```python
from build123d import *

# Parameters (mm, degrees)
SKETCH1_W             = 96
SKETCH1_H             = 12
BOSS_EXTRUDE1_DEPTH   = 30
SKETCH1_3_R           = 7.5
BOSS_EXTRUDE2_DEPTH   = 6
BOSS_EXTRUDE3_DEPTH   = 20
BOSS_EXTRUDE4_DEPTH   = 7
F_8_0MM_DOWEL_HOLE1_D = 8
F_8_0MM_DOWEL_HOLE2_D = 8


with BuildPart() as part:
    # Sketch1 → Boss-Extrude1 (new body)
    with BuildSketch(Plane.XY):
        with Locations((0, 6)):
            Rectangle(SKETCH1_W, SKETCH1_H)
    extrude(amount=BOSS_EXTRUDE1_DEPTH)

    # Sketch1_3 → Boss-Extrude2 (add)
    with BuildSketch(Plane.XY):
        with BuildLine():
            ThreePointArc((-15, 56), (0, 41), (15, 56))
            Line((15, 56), (15, 46))
            Line((15, 46), (27, 46))
            ThreePointArc((27, 46), (34.864825613, 27.37239229), (48, 12))
            Line((48, 12), (-48, 12))
            ThreePointArc((-48, 12), (-34.864825613, 27.37239229), (-27, 46))
            Line((-27, 46), (-15, 46))
            Line((-15, 46), (-15, 56))
        make_face()
        with Locations((0, 27)):
            Circle(SKETCH1_3_R, mode=Mode.SUBTRACT)
    extrude(amount=BOSS_EXTRUDE2_DEPTH)

    # Sketch1_4 → Boss-Extrude3 (add)
    with BuildSketch(Plane.XY):
        Polygon((-27, 46), (-15, 46), (-15, 56), (-15, 66), (-27, 66), align=None)
        Polygon((15, 46), (15, 56), (15, 66), (27, 66), (27, 46), align=None)
    extrude(amount=BOSS_EXTRUDE3_DEPTH)

    # Sketch2 → Boss-Extrude4 (add)
    with BuildSketch(Plane(origin=(-15, 0, 0), x_dir=(0, 0, -1), z_dir=(1, 0, 0))):
        with BuildLine():
            Line((-20, 46), (-6, 46))
            Line((-6, 46), (-6, 12))
            Line((-6, 12), (-30, 12))
            ThreePointArc((-30, 12), (-22.675193853, 28.316233486), (-20, 46))
        make_face()
    boss_extrude4 = extrude(amount=-BOSS_EXTRUDE4_DEPTH)

    # Mirror1: Boss-Extrude4 across plane
    add(boss_extrude4.mirror(Plane(origin=(0, 0, 0), x_dir=(0, 0, 1), z_dir=(1, 0, 0))))

    # 8.0mm Dowel Hole1 (through all)
    with Locations(Plane(origin=(-27, 56, 10), x_dir=(0, -1, 0), z_dir=(-1, 0, 0))):
        with Locations((0, 0)):
            Hole(F_8_0MM_DOWEL_HOLE1_D / 2)

    # 8.0mm Dowel Hole2 (through all)
    with Locations(Plane(origin=(-32.5, 12, 18), x_dir=(0, 0, 1), z_dir=(0, 1, 0))):
        with Locations((0, 0), (0.381139368, 64.99888255)):
            Hole(F_8_0MM_DOWEL_HOLE2_D / 2)


solid = part.part
```
Can you work these out from the model? Positions are in its coordinate system, mm. A direction names the side the tool comes from. Round coordinates to 2 decimals unless told otherwise and drop trailing zeros. Loops run counter-clockwise (first coordinate to the right, second up) from the corner with the lowest first, then second, coordinate; pieces in that order, holes last. Notation, with made-up numbers: M 23.25,11 L 71.25,11 A19 ccw 71.25,19 Z; hole C -15.5,-30.5 d6. An arc over 180 degrees is marked long. Answer as a JSON object with one key per item and string values. Group by question number.
Q1. Imagine slicing it at B-B, the plane x = 0. Please give me the cut outline in (y, z), then the cut area to 3 significant figures.
Q2. We'd pull the mould along Y, two halves only. Please class faces 1 (the flat face through (0, 12, 18)), 2 (the flat face through (-22, 29, 15)), 3 (the flat face through (-1, 0, 15)), 4 (the flat face through (-21, 56, 20)): +Y half, -Y half, draft (parallel to the pull), parting line (faces both ways), or undercut.
Q3. Imagine slicing it at A-A, the plane z = 10. Please give me the cut outline in (x, y), then the cut area to 3 significant figures.
Q4. Will these pins go through, and if not, where does the flat tip stop? pin 1 (13 mm diameter, centred on x = 22, y = 58, fed in from +Z); pin 2 (1.5 mm diameter, centred on x = -34, z = 13, fed in from +Y); pin 3 (7 mm diameter, centred on y = 27, z = 16.5, fed in from +X).
Q5. Imagine slicing it at C-C, the plane y = 31. Please give me the cut outline in (x, z).
Q6. On a 3-axis mill with a long thin cutter (end or side, diameter ignored), from which of +Z, -Z, +X, -X, +Y, -Y can I reach the whole of each face in a straight line? I mean faces 5 (the cylindrical face through (0, 41, 3)), 6 (the flat face through (4, 34, 6)), 7 (the flat face through (-38, 12, 18)), 8 (the flat face through (21, 56, 20)). Say none if no direction works.
Q7. Please list where these lines run through material, in increasing order: L1, parallel to Y at x = -20.75, z = 10; L2, parallel to X at y = 19, z = 14; L3, parallel to X at y = 10, z = 20.5.
Q8. Imagine slicing it at D-D, the plane y = 5. Please give me the cut outline in (x, z).
Findings:
{
 "1": {"outline": "M 0,0 L 19.5,0 L 19.5,6 L 12,6 L 12,30 L 0,30 Z; M 34.5,0 L 41,0 L 41,6 L 34.5,6 Z", "area": "444 mm2"},
 "2": {"face 1": "+Y half", "face 2": "undercut", "face 3": "-Y half", "face 4": "draft"},
 "3": {"outline": "M -48,0 L 48,0 L 48,12 L 22,12 L 22,46 L 27,46 L 27,52 L 15,52 L 15,12 L -15,12 L -15,52 L -27,52 L -27,46 L -22,46 L -22,12 L -48,12 Z; M -27,60 L -15,60 L -15,66 L -27,66 Z; M 15,60 L 27,60 L 27,66 L 15,66 Z", "area": "1,920 mm2"},
 "4": {"pin 1": "stops at z = 20", "pin 2": "stops at y = 12", "pin 3": "stops at x = 22"},
 "5": {"outline": "M -32.78,0 L -6.34,0 L -6.34,6 L -15,6 L -15,21.95 L -22,21.95 L -22,6 L -32.78,6 Z; M 6.34,0 L 32.78,0 L 32.78,6 L 22,6 L 22,21.95 L 15,21.95 L 15,6 L 6.34,6 Z"},
 "6": {"face 5": "+Z, -Z, +Y", "face 6": "+Z, +Y", "face 7": "+Z, -X", "face 8": "+Z, +X, -X, +Y"},
 "7": {"L1": "y = 0 to 52, 60 to 66", "L2": "x = -22 to -15, 15 to 22", "L3": "x = -48 to -35.62, -29.38 to 29.11, 35.89 to 48"},
 "8": {"outline": "M -48,0 L 48,0 L 48,30 L -48,30 Z; hole C -32.5,18 d8; hole C 32.5,18.38 d8"}
}
